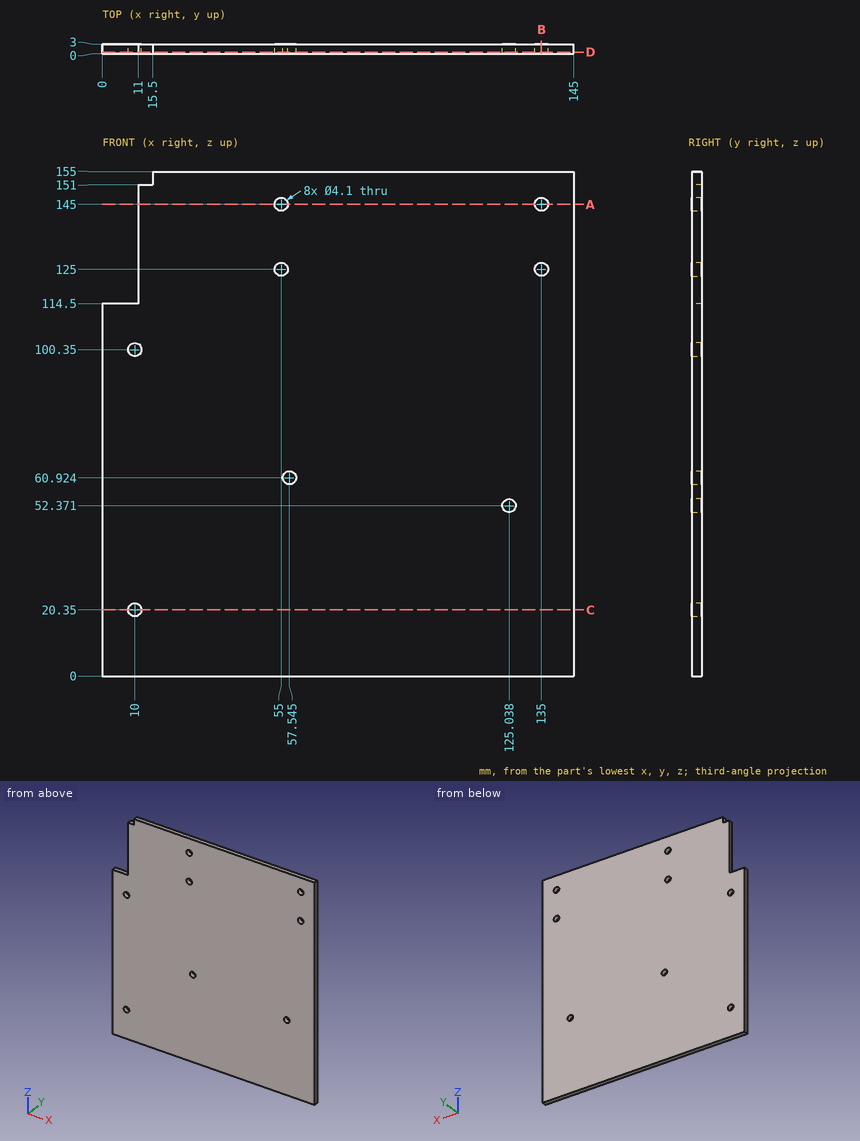
Job drawing, mm, ordinate dimensions from the low corner. One solid piece. Give positions to 0.01 mm unless a question says otherwise; leave off trailing zeros. Order: outer loops, then holes, each group sorted by start corner. A loop starts at its lowest first (then second) coordinate and runs counter-clockwise, first axis right, second up. Notation, with made-up numbers: (7.25, 3.5) - (27.25, 3.5) arc R11 cw to (27.25, 15.5) - close; hole circle Ø3 at (-37.5, -14). An arc over 180 degrees is marked (long way). One line per question, with ' | ' between items.
1. Drill centre lines: probe 1 along X at (y, z) = (0.95, 145); probe 2 along X at (y, z) = (1, 135.5); probe 3 along X at (y, z) = (2, 100.35). Where is each one in solid material? Low to high.
Filled in:
probe 1: 11 to 52.95, 57.05 to 132.95, 137.05 to 145 | probe 2: 11 to 145 | probe 3: 0 to 7.95, 12.05 to 145
2. Band-saw the part on C-C on z = 20.35. List the corners of the cut face in (x, y).
Filled in:
outline: (0, 0) - (7.95, 0) - (7.95, 3) - (0, 3) - close; (12.05, 0) - (145, 0) - (145, 3) - (12.05, 3) - close
3. Band-saw the part on D-D on y = 0.5. Give the number of separate pieces and of enclosed holes in the cut face, then the cut area to 3 significant figures.
Filled in:
separate pieces: 1 | enclosed holes: 8 | area: 21,900 mm²
4. Band-saw the part on B-B on x = 135. List the corners of the cut face in (y, z).
Filled in:
outline: (0, 0) - (3, 0) - (3, 122.95) - (0, 122.95) - close; (0, 127.05) - (3, 127.05) - (3, 142.95) - (0, 142.95) - close; (0, 147.05) - (3, 147.05) - (3, 155) - (0, 155) - close
5. Drop flat-ended pins along their axis: P1, Ø3.5, axis at x = 135, z = 145, coming from the +Y side (3 decimals); P2, Ø0.9, axis at y = 2, z = 152.5, coming from the -X side; P3, Ø0.9, axis at y = 1, z = 135.5, coming from the -X side. Give the stop position or say it passes through.
Filled in:
P1: through | P2: x = 15.5 | P3: x = 11
6. Band-saw the part on A-A on z = 145. List the corners of the cut face in (x, y).
Filled in:
outline: (11, 0) - (52.95, 0) - (52.95, 3) - (11, 3) - close; (57.05, 0) - (132.95, 0) - (132.95, 3) - (57.05, 3) - close; (137.05, 0) - (145, 0) - (145, 3) - (137.05, 3) - close
